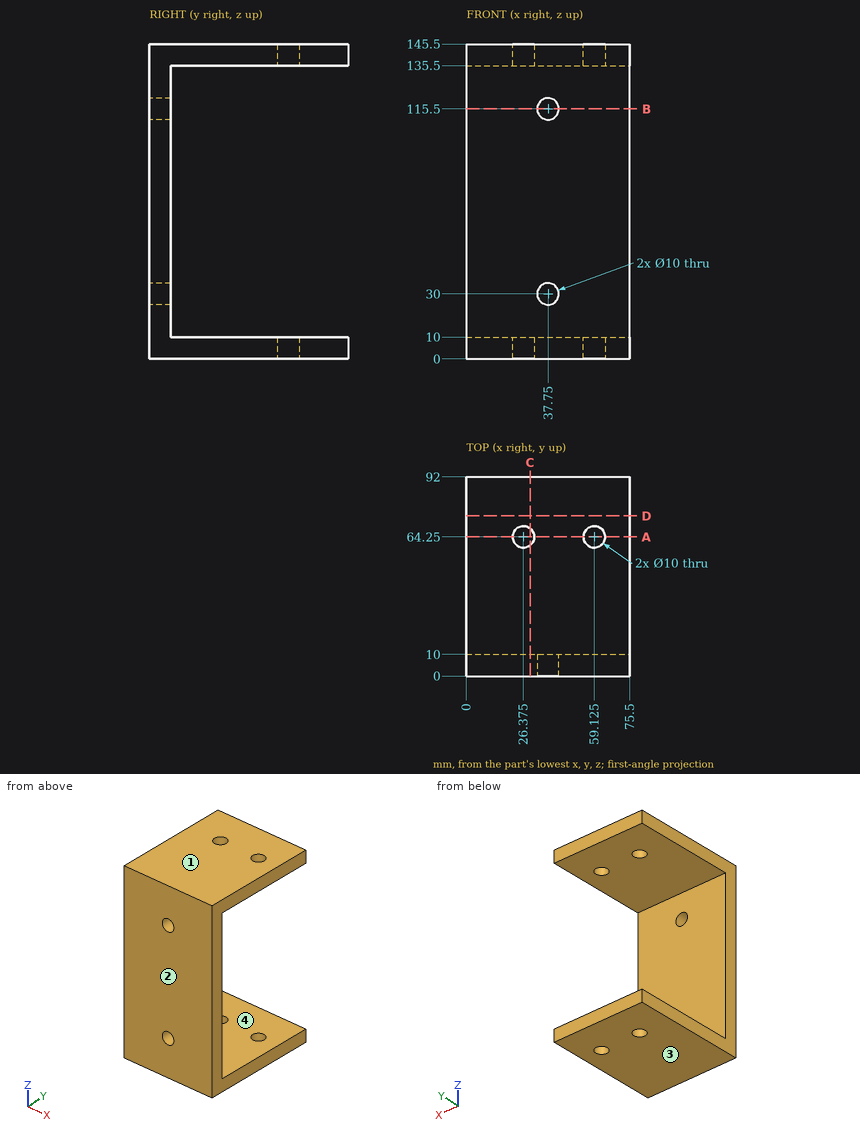
Job drawing, mm, ordinate dimensions from the low corner. One solid piece. Round coordinates to 2 decimals unless told otherwise and drop trailing zeros. Loops run counter-clockwise (first coordinate to the right, second up) from the corner with the lowest first, then second, coordinate; pieces in that order, holes last. Notation, with made-up numbers: (-36.5, -39) -> (-11.5, -39) arc R16 ccw to (-11.5, -29) -> close; hole circle Ø8 at (31.25, -36). An arc over 180 degrees is marked (long way). Use CSV: the item, a comma, the result in double quotes. Start each with the question number.
Q1. Mould opens along Z. For the marked faces 1, 2, 3 and 4 say: +Z half, -Z half, draft (parallel to the pull), parting line (faces both ways), or undercut.
Q2. Flat gauge pins, fed straight in: pin 1 Ø2 at (x, y) = (52, 76.5) entering from -Z; pin 2 Ø4 at (x, z) = (12.5, 74.5) entering from +Y; pin 3 Ø9 at (x, y) = (26.375, 64.25) entering from -Z. Where does each tip first touch, or does it go through?
Q3. Saw through at C-C on x = 29.5. Give the cut face in (y, z).
Q4. Saw through at A-A on y = 64.25. Give the cut face in (x, z) (3 decimals).
Q5. Saw through at B-B on z = 115.5. Give the cut face in (x, y), and give its area (3 significant figures).
Q6. Drill centre lines: L1, parallel to Z at x = 37.75, y = 5.75; L2, parallel to X at y = 64.25, z = 6.5 (3 decimals); L3, parallel to Z at x = 65, y = 46. Where is each one in solid material? Low to high.
Q7. Saw through at D-D on y = 74. Give the cut face in (x, z), and give its area (3 significant figures).
Solutions:
1,face 1,"+Z half"
1,face 2,"draft"
1,face 3,"-Z half"
1,face 4,"undercut"
2,pin 1,"stops at z = 0"
2,pin 2,"stops at y = 10"
2,pin 3,"passes through"
3,outline,"(0, 0) -> (60.35, 0) -> (60.35, 10) -> (10, 10) -> (10, 135.5) -> (60.35, 135.5) -> (60.35, 145.5) -> (0, 145.5) -> close; (68.15, 0) -> (92, 0) -> (92, 10) -> (68.15, 10) -> close; (68.15, 135.5) -> (92, 135.5) -> (92, 145.5) -> (68.15, 145.5) -> close"
4,outline,"(0, 0) -> (21.375, 0) -> (21.375, 10) -> (0, 10) -> close; (0, 135.5) -> (21.375, 135.5) -> (21.375, 145.5) -> (0, 145.5) -> close; (31.375, 0) -> (54.125, 0) -> (54.125, 10) -> (31.375, 10) -> close; (31.375, 135.5) -> (54.125, 135.5) -> (54.125, 145.5) -> (31.375, 145.5) -> close; (64.125, 0) -> (75.5, 0) -> (75.5, 10) -> (64.125, 10) -> close; (64.125, 135.5) -> (75.5, 135.5) -> (75.5, 145.5) -> (64.125, 145.5) -> close"
5,outline,"(0, 0) -> (32.75, 0) -> (32.75, 10) -> (0, 10) -> close; (42.75, 0) -> (75.5, 0) -> (75.5, 10) -> (42.75, 10) -> close"
5,area,"655 mm^2"
6,L1,"z = 0 to 25, 35 to 110.5, 120.5 to 145.5"
6,L2,"x = 0 to 21.375, 31.375 to 54.125, 64.125 to 75.5"
6,L3,"z = 0 to 10, 135.5 to 145.5"
7,outline,"(0, 0) -> (75.5, 0) -> (75.5, 10) -> (0, 10) -> close; (0, 135.5) -> (75.5, 135.5) -> (75.5, 145.5) -> (0, 145.5) -> close"
7,area,"1,510 mm^2"
